Source: CAD feature listing. Evaluate the final solid. Frame: model axes, mm. A direction names the side the tool comes from. Round coordinates to 2 decimals unless told otherwise and drop trailing zeros. Order: outer loops, then holes, each group sorted by start corner. A loop starts at its lowest first (then second) coordinate and runs counter-clockwise, first axis right, second up. Notation, with made-up numbers: (45.25, 70) - (51.25, 70) arc R23 ccw to (51.25, 91) - close; hole circle Ø1 at (37, -20.5). An arc over 180 degrees is marked (long way). Use one line per item in the form item = value. Start each with the question number.
Q1. Cut plane B-B, the plane z = 1.4. Return the cut outline in (x, y), and give its area (3 significant figures).
Q2. Set-up query: faces 4 (the flat face through (30, 80, 1)), 5 (the flat face through (-1, 20, 1)), 6 (the flat face through (-3, 10, 1)). Return all of +Z, -Z, +X, -X, +Y, -Y with unobstructed straight access to the full face (end or side cutting, diameter ignored); none if empty.
Q3. Cut plane C-C, the plane x = 31. Return the cut outline in (y, z).
Q4. Draft query along Y for faces 1 (the flat face through (47, 80, 1)), 2 (the flat face through (-3, 50, 1)), 3 (the flat face through (33, 66, 1)). Return one class per face: released by +Y, released by -Y, zero draft, split by the parting line, or undercut.
Q5. Ray query, line 1 (X direction, y = 75.5, z = 0.9); line 2 (Y direction, x = 43, z = 1.9); line 3 (Y direction, x = 42, z = 1.2). Return the intervals inside material, ascending. Write a range as [from, to].
Q6. Pin query (flat end, axial travel): pin 1 Ø1.5 at (y, z) = (73, 1) entering from -X; pin 2 Ø5 at (x, y) = (29.5, 72.5) entering from -Z; pin 3 Ø1.5 at (x, z) = (31, 2) entering from -Y. Return the tip coordinate at first contact, or that it passes through.
Q7. Cut plane A-A, the plane y = 62. Return the cut outline in (x, z).
Q8. Cut plane D-D, the plane x = 37. Return the cut outline in (y, z), and give its area (3 significant figures).
from build123d import *

# Parameters (mm, degrees)
SKETCH1_W           = 3
SKETCH1_H           = 20
BOSS_EXTRUDE1_DEPTH = 3


with BuildPart() as part:
    # Sketch1 → Boss-Extrude1 (new body)
    with BuildSketch(Plane.XY):
        Polygon((-3, 60), (-3, 40), (0, 40), (0, 20), (-3, 20), (-3, 0), (0, 0), (45, 54.545454545), (33, 54.545454545), (33, 77.545454545), (45, 77.545454545), (45, 60), (48, 60), (48, 80), (45, 80), (45, 90), (15, 90), (-3, 90), (-3, 80), (0, 80), (0, 60), align=None)
        with Locations((30.5, 70)):
            Rectangle(SKETCH1_W, SKETCH1_H, mode=Mode.SUBTRACT)
    extrude(amount=BOSS_EXTRUDE1_DEPTH)


solid = part.part
Completed:
q1.outline = (-3, 0) - (0, 0) - (45, 54.55) - (33, 54.55) - (33, 77.55) - (45, 77.55) - (45, 60) - (48, 60) - (48, 80) - (45, 80) - (45, 90) - (-3, 90) - (-3, 80) - (0, 80) - (0, 60) - (-3, 60) - (-3, 40) - (0, 40) - (0, 20) - (-3, 20) - close; hole (29, 60) - (32, 60) - (32, 80) - (29, 80) - close
q1.area = 2,700 mm2
q2.face_4 = +Z, -Z
q2.face_5 = +Z, -Z, -X
q2.face_6 = +Z, -Z, -X, +Y, -Y
q3.outline = (37.58, 0) - (60, 0) - (60, 3) - (37.58, 3) - close; (80, 0) - (90, 0) - (90, 3) - (80, 3) - close
q4.face_1 = released by +Y
q4.face_2 = zero draft
q4.face_3 = undercut
q5.line_1 = [0, 29], [32, 33], [45, 48]
q5.line_2 = [52.12, 54.55], [77.55, 90]
q5.line_3 = [50.91, 54.55], [77.55, 90]
q6.pin_1 = 0
q6.pin_2 = 0
q6.pin_3 = 36.67
q7.outline = (0, 0) - (29, 0) - (29, 3) - (0, 3) - close; (32, 0) - (33, 0) - (33, 3) - (32, 3) - close; (45, 0) - (48, 0) - (48, 3) - (45, 3) - close
q8.outline = (44.85, 0) - (54.55, 0) - (54.55, 3) - (44.85, 3) - close; (77.55, 0) - (90, 0) - (90, 3) - (77.55, 3) - close
q8.area = 66.5 mm2
